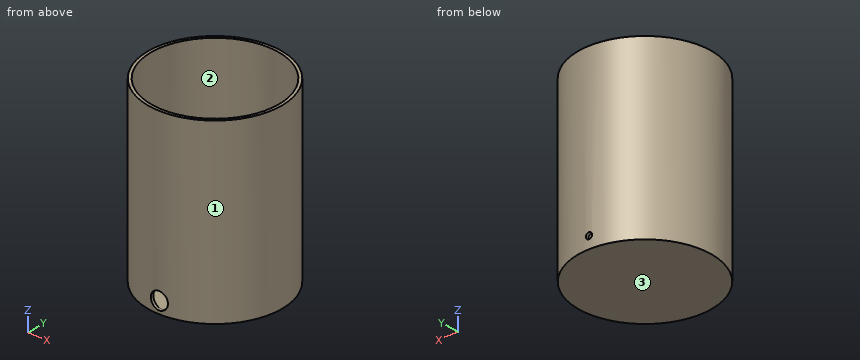
from build123d import *

# Parameters (mm, degrees)
F0_R     = 285.75
F1_DEPTH = 762
F2_T     = -12.7
F3_R     = 36.5125
F4_DEPTH = 327.66
F5_R     = 13.335
F6_DEPTH = 345.44


with BuildPart() as f1:
    # F0 (on Top) → F1 (new body)
    with BuildSketch(Plane.XY):
        Circle(F0_R)
    extrude(amount=F1_DEPTH)

    # F2
    f2_openings = [f1.faces().sort_by_distance(p)[0] for p in [
        (0, 0, 762),
    ]]
    offset(amount=F2_T, openings=f2_openings)

    # F3 (on Front) → F4 (cut)
    with BuildSketch(Plane.XZ):
        with Locations((0, 50.8)):
            Circle(F3_R)
    extrude(amount=F4_DEPTH, mode=Mode.SUBTRACT)

    # F5 (on Front) → F6 (cut)
    with BuildSketch(Plane.XZ):
        with Locations((0, 50.8)):
            Circle(F5_R)
    extrude(amount=-F6_DEPTH, mode=Mode.SUBTRACT)


solid = f1.part
CAD build for the part. Positions are in the model's coordinates, mm. Face numbers are marked on the shaded views. Round coordinates to 2 decimals unless told otherwise and drop trailing zeros. Loops run counter-clockwise (first coordinate to the right, second up) from the corner with the lowest first, then second, coordinate; pieces in that order, holes last.
(1) Two-plate mould, pull along Y, no slides. Class the marked faces 1, 2 and 3: +Y half, -Y half, draft (parallel to the pull), parting line (faces both ways), or undercut.
(2) Drop flat-ended pins along their axis: pin 1 (1.5 mm diameter, centred on y = 50.5, z = 170.5, fed in from +X); pin 2 (8 mm diameter, centred on y = -202.5, z = 364.5, fed in from -X); pin 3 (6 mm diameter, centred on y = -34.5, z = 233.5, fed in from +X); pin 4 (24 mm diameter, centred on x = 0, z = 50.8, fed in from +Y). Give the stop position or say it passes through.
(3) Cut at A-A (x = 0). State how many separate pieces and enclosed holes the cut face has, plus the area to 3 significant figures.
(4) Wall check: line 1 along Z through (x, y) = (0, 282) (3 decimals); line 2 along Y through (x, z) = (0, 387); line 3 along Z through (x, y) = (0, -274.5). Give the ranges that are in metal, low to high.
(5) Cut at C-C (y = 0). Give the cut face in (x, z), plus the area to 3 significant figures.
(6) Cut at D-D (x = -140). Give the cut face in (y, z), plus the area to 3 significant figures.
Findings below:
1. face 1: parting line
1. face 2: undercut
1. face 3: draft
2. pin 1: stops at x = 281.39
2. pin 2: stops at x = -205.55
2. pin 3: stops at x = 284.01
2. pin 4: passes through
3. separate pieces: 3
3. enclosed holes: 0
3. area: 25,000 mm2
4. line 1: z = 0 to 37.465, 64.135 to 762
4. line 2: y = -285.75 to -273.05, 273.05 to 285.75
4. line 3: z = 0 to 14.29, 87.31 to 762
5. outline: (-285.75, 0) - (285.75, 0) - (285.75, 762) - (273.05, 762) - (273.05, 12.7) - (-273.05, 12.7) - (-273.05, 762) - (-285.75, 762) - close
5. area: 26,300 mm2
6. outline: (-249.1, 0) - (249.1, 0) - (249.1, 762) - (234.43, 762) - (234.43, 12.7) - (-234.43, 12.7) - (-234.43, 762) - (-249.1, 762) - close
6. area: 28,300 mm2
